The listing builds one solid part. Answer for the finished solid, in the listing's coordinates (mm). Coordinates: 2 decimals unless noted, no trailing zeros. Order: outer loops, then holes, each group sorted by start corner. A loop starts at its lowest first (then second) coordinate and runs counter-clockwise, first axis right, second up. Notation, with made-up numbers: (-24.5, 77) -> (-2.5, 77) arc R18 ccw to (-2.5, 83) -> close; hole circle Ø11 at (82.25, 14.5). An arc over 180 degrees is marked (long way). Answer in a Markdown table with one row per item.
```python
from build123d import *

# Parameters (mm, degrees)
SKETCH1_W           = 15.7
SKETCH1_H           = 6.33
BOSS_EXTRUDE1_DEPTH = 2.95


with BuildPart() as part:
    # Sketch1 → Boss-Extrude1 (new body)
    with BuildSketch(Plane.XY):
        with BuildLine():
            Line((-56.418907266, 103.171587302), (-53.918907266, 103.171587302))
            Line((-53.918907266, 103.171587302), (-53.918907266, 108.801587302))
            Line((-53.918907266, 108.801587302), (-38.918907266, 108.801587302))
            Line((-38.918907266, 108.801587302), (-38.918907266, 103.171587302))
            Line((-38.918907266, 103.171587302), (-36.418907266, 103.171587302))
            ThreePointArc((-36.418907266, 103.171587302), (0.378461485, 91.312248832), (38.831092734, 87.301587302))
            Line((38.831092734, 87.301587302), (38.831092734, -112.698412698))
            Line((38.831092734, -112.698412698), (-131.668907266, -112.698412698))
            Line((-131.668907266, -112.698412698), (-131.668907266, 87.301587302))
            ThreePointArc((-131.668907266, 87.301587302), (-93.216276016, 91.312248832), (-56.418907266, 103.171587302))
        make_face()
        with Locations((-46.418907266, 84.136587302)):
            Rectangle(SKETCH1_W, SKETCH1_H, mode=Mode.SUBTRACT)
    extrude(amount=BOSS_EXTRUDE1_DEPTH)


solid = part.part
```
(1) Flat-ended cylindrical pins translate along their axes: pin 1 (1.5 mm diameter, centred on y = 105.5, z = 2, fed in from -X); pin 2 (0.8 mm diameter, centred on x = -55.5, z = 1, fed in from +Y); pin 3 (10 mm diameter, centred on x = -14.5, y = -14, fed in from -Z). Find the tip coordinate at first contact, or state that the pin passes through.
Check values:
| item | result |
|---|---|
| pin 1 | x = -53.92 |
| pin 2 | y = 103.17 |
| pin 3 | z = 0 |
(2) A cutting plane is placed at C-C, the plane x = -68.5. Determine the outline of the cut face in (y, z), then the cut area to 3 significant figures.
Check values:
| item | result |
|---|---|
| outline | (-112.7, 0) -> (98.34, 0) -> (98.34, 2.95) -> (-112.7, 2.95) -> close |
| area | 623 mm² |
(3) Find the intervals of material crossed by line 1 along Y through (x, z) = (-50, 2.05); line 2 along Y through (x, z) = (-92.5, 1.85); line 3 along Y through (x, z) = (-18.5, 1.8), in increasing order. Write a range as from..to.
Check values:
| item | result |
|---|---|
| line 1 | -112.7..80.97, 87.3..108.8 |
| line 2 | -112.7..91.46 |
| line 3 | -112.7..96.34 |
(4) A cutting plane is placed at A-A, the plane z = 1.55. Determine the outline of the cut face in (x, y), then the cut area to 3 significant figures.
Check values:
| item | result |
|---|---|
| outline | (-131.67, -112.7) -> (38.83, -112.7) -> (38.83, 87.3) arc R186.34 cw to (-36.42, 103.17) -> (-38.92, 103.17) -> (-38.92, 108.8) -> (-53.92, 108.8) -> (-53.92, 103.17) -> (-56.42, 103.17) arc R186.34 cw to (-131.67, 87.3) -> close; hole (-54.27, 80.97) -> (-38.57, 80.97) -> (-38.57, 87.3) -> (-54.27, 87.3) -> close |
| area | 35,200 mm² |
(5) A cutting plane is placed at B-B, the plane x = -106.5. Determine the outline of the cut face in (y, z).
Check values:
| item | result |
|---|---|
| outline | (-112.7, 0) -> (89.01, 0) -> (89.01, 2.95) -> (-112.7, 2.95) -> close |
